Source: three-view drawing plus pictorial views. Frame: mm from the lowest corner of the part. Give positions to 0.01 mm unless a question says otherwise; leave off trailing zeros. Write each loop counter-clockwise with the first axis right and the second up, starting at its lowest first coordinate (ties: lowest second). Pieces come first, ordered by that corner, then holes.
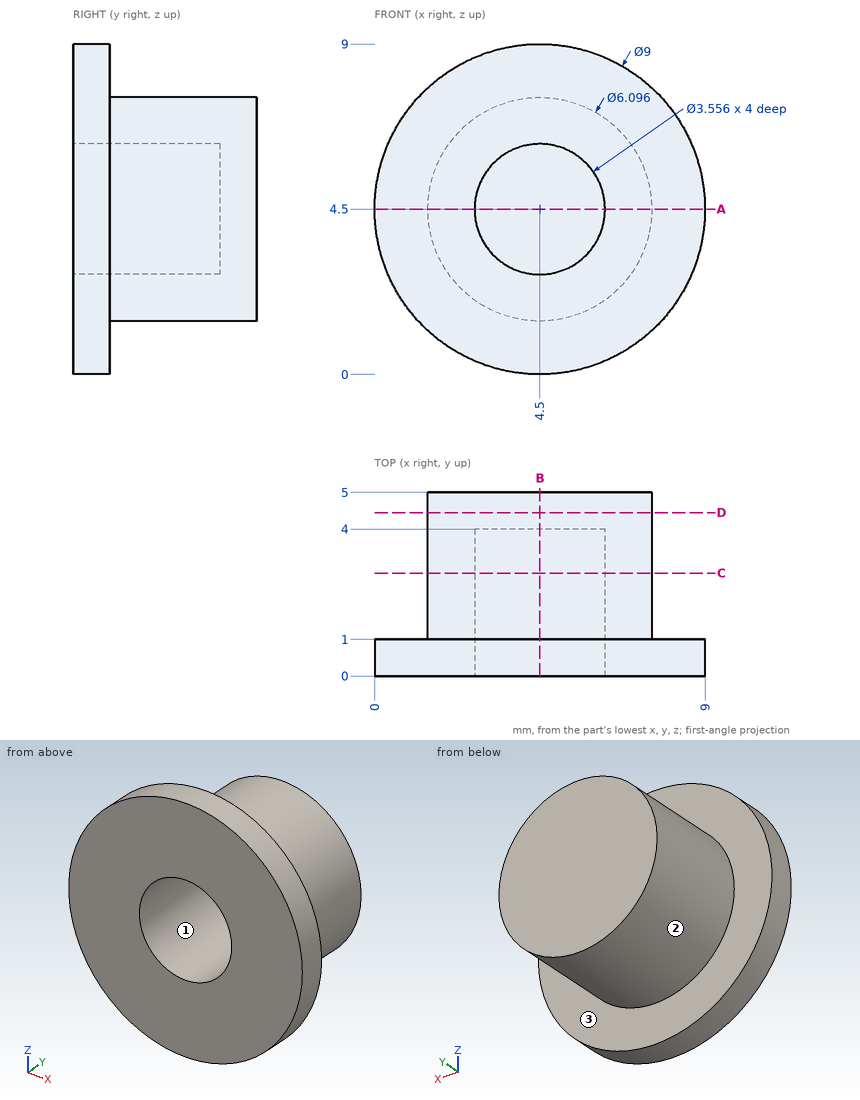
Q1. Section A-A on z = 4.5. Output: boundary loops of the cut face in (x, y).
Filled sheet:
outline: (0, 0) - (2.72, 0) - (2.72, 4) - (6.28, 4) - (6.28, 0) - (9, 0) - (9, 1) - (7.55, 1) - (7.55, 5) - (1.45, 5) - (1.45, 1) - (0, 1) - close
Q2. Section D-D on y = 4.45. Output: boundary loops of the cut face in (x, z).
Filled sheet:
outline: circle Ø6.1 at (4.5, 4.5)
Q3. Pin query (flat end, axial travel): P1, Ø2, axis at x = 7.5, y = 4, coming from the -Z side; P2, Ø1.1, axis at x = 3.5, z = 5, coming from the -Y side. Return the tip coordinate at first contact, or that it passes through.
Filled sheet:
P1: stops at z = 2.2
P2: stops at y = 4
Q4. Pull-direction query (X, two-part tool) for the marked faces 1, 2 and 3; classes: released by +X, released by -X, zero draft, split by the parting line, or undercut.
Filled sheet:
face 1: undercut
face 2: split by the parting line
face 3: zero draft
Q5. Ray query, line 1 along Z through (x, y) = (4.5, 1.25); line 2 along Z through (x, y) = (4.5, 0.95); line 3 along Y through (x, z) = (7.5, 1.25). Return the intervals inside material, ascending.
Filled sheet:
line 1: z = 1.45 to 2.72, 6.28 to 7.55
line 2: z = 0 to 2.72, 6.28 to 9
line 3: y = 0 to 1
Q6. Section C-C on y = 2.8. Output: boundary loops of the cut face in (x, z), plus the area to 3 significant figures.
Filled sheet:
outline: circle Ø6.1 at (4.5, 4.5); hole circle Ø3.56 at (4.5, 4.5)
area: 19.3 mm2
Q7. Section B-B on x = 4.5. Output: boundary loops of the cut face in (y, z), plus the area to 3 significant figures.
Filled sheet:
outline: (0, 0) - (1, 0) - (1, 1.45) - (5, 1.45) - (5, 7.55) - (1, 7.55) - (1, 9) - (0, 9) - (0, 6.28) - (4, 6.28) - (4, 2.72) - (0, 2.72) - close
area: 19.2 mm2
